Geometry check sheet. Reference: the model listing, model coordinates, mm. A direction names the side the tool comes from. Coordinates: 2 decimals unless noted, no trailing zeros. Loops run counter-clockwise (first coordinate to the right, second up) from the corner with the lowest first, then second, coordinate; pieces in that order, holes last. Notation, with made-up numbers: (48, 86.5) -> (89, 86.5) arc R19 cw to (89, 112.5) -> close; hole circle Ø2 at (69, 5.25). An arc over 180 degrees is marked (long way). Answer as a JSON object with one key per item and string values.
from build123d import *

# Parameters (mm, degrees)
F0_W     = 21.5
F0_H     = 21.4
F1_DEPTH = 1
F0_H_2   = 4
F2_DEPTH = 3
F4_D     = 2.85
F5_R     = 2


with BuildPart() as f1:
    # F0 (on Top) → F1 (new body)
    with BuildSketch(Plane.XY):
        Rectangle(F0_W, F0_H)
    extrude(amount=F1_DEPTH)

    # F0 (on Top) → F2 (join)
    with BuildSketch(Plane.XY):
        with Locations((0, 12.7)):
            Rectangle(F0_W, F0_H_2)
        with Locations((0, -12.7)):
            Rectangle(F0_W, F0_H_2)
    extrude(amount=F2_DEPTH)

    # F4 (through all)
    with Locations(Plane.YZ.offset(10.75)):
        with Locations((12.7, 2), (-12.7, 2)):
            Hole(F4_D / 2)

    # F5
    f5_edges = [f1.edges().sort_by_distance(p)[0] for p in [
        (0, 14.7, 0),
        (0, -14.7, 0),
    ]]
    fillet(f5_edges, radius=F5_R)


solid = f1.part
1. Depth check by flat-ended pin: P1, Ø6.5, axis at x = 0, y = 0, coming from the +Z side; P2, Ø1, axis at x = 0, z = 0.5, coming from the +Y side. Enter the tip coordinate at first touch or a pass-through.
Evaluation:
{"P1": "stops at z = 1", "P2": "stops at y = 14.43"}
2. Mould release check, pull along Y, two halves, no side actions. Record for faces 1 (the face through (-0.2, -14.7, 2.5)), 2 (the face through (0.15, 14.1, 0.57)), 3 (the face through (0, -11, 3)), 4 (the face through (0, 10.7, 2)): released by +Y, released by -Y, zero draft, split by the parting line, or undercut.
Evaluation:
{"face 1": "released by -Y", "face 2": "released by +Y", "face 3": "zero draft", "face 4": "undercut"}
3. Thickness scan on probe 1 along Y at (x, z) = (-3.25, 2) (3 decimals); probe 2 along Y at (x, z) = (-10, 2.6); probe 3 along Z at (x, y) = (-2.75, -12.75). Record the ranges inside material, lowest first. Write a range as from..to.
Evaluation:
{"probe 1": "y = -14.7..-14.125, -11.275..-10.7, 10.7..11.275, 14.125..14.7", "probe 2": "y = -14.7..-13.99, -11.41..-10.7, 10.7..11.41, 13.99..14.7", "probe 3": "z = 0..0.58"}
4. Section check B-B, the plane y = -1.25. Record the boundary of the cut face in (x, z), then the cut area to 3 significant figures.
Evaluation:
{"outline": "(-10.75, 0) -> (10.75, 0) -> (10.75, 1) -> (-10.75, 1) -> close", "area": "21.5 mm^2"}
5. Tool access check on faces 5 (the face through (-10.75, -0.1, 0.6)), 6 (the face through (0, 0, 1)). Record the directions out of +Z, -Z, +X, -X, +Y, -Y that give a thin tool (end or side, any length) a straight path to the whole face; none if there is none.
Evaluation:
{"face 5": "+Z, -Z, -X, +Y, -Y", "face 6": "+Z, +X, -X"}
6. Section check A-A, the plane x = 7. Record the boundary of the cut face in (y, z) (3 decimals), then the cut area to 3 significant figures.
Evaluation:
{"outline": "(-14.7, 2) arc R2 ccw to (-12.7, 0) -> (12.7, 0) arc R2 ccw to (14.7, 2) -> (14.7, 3) -> (13.715, 3) arc R1.425 cw (long way) to (11.685, 3) -> (10.7, 3) -> (10.7, 1) -> (-10.7, 1) -> (-10.7, 3) -> (-11.685, 3) arc R1.425 cw (long way) to (-13.715, 3) -> (-14.7, 3) -> close", "area": "32.1 mm^2"}
